The model under review builds one solid part; all positions refer to its coordinate system, in mm. Face numbers are marked on the shaded views. Round coordinates to 2 decimals unless told otherwise and drop trailing zeros. Write each loop counter-clockwise with the first axis right and the second up, starting at its lowest first coordinate (ties: lowest second). Pieces come first, ordered by that corner, then holes.
Item 1: Draft analysis for pull direction Z (two halves, no side actions). For the marked faces 1 and 2, state which applies: +Z half, -Z half, draft (parallel to the pull), parting line (faces both ways), or undercut.
Item 2: To check wall thickness, follow L1, parallel to X at y = 8.6, z = -4; L2, parallel to Z at x = 1, y = 7.35; L3, parallel to X at y = 4.3, z = 0. State the ranges of each line that lie inside material, in increasing order.
Item 3: Add section A-A (y = 7.15). Give the boundary of the cut face in (x, z), plus the area to 3 significant figures.
Item 4: Clearance check with flat-ended pins moving along their axes: pin 1 Ø2.5 at (x, z) = (-0.5, 1) entering from +Y; pin 2 Ø1 at (x, z) = (2.5, 0.5) entering from -Y; pin 3 Ø5 at (x, z) = (-1.5, 2) entering from +Y; pin 4 Ø2 at (y, z) = (5, 1.5) entering from -X. State where each tip first meets the part, or that it passes through.
```python
from build123d import *

# Parameters (mm, degrees)
EXTRUDE_1_DEPTH          = 0.6
EXTRUDE_1_DEPTH_BACK     = 6
SKETCH_5_R               = 0.31
SKETCH_7_R               = 0.28
CUT_EXTRUDE_2_DEPTH      = 16.448840302
CUT_EXTRUDE_3_DEPTH      = 10
CUT_EXTRUDE_3_DEPTH_BACK = 10


with BuildPart() as part:
    # Sketch 2 → Revolve 1 (revolve)
    with BuildSketch(Plane.XY, mode=Mode.PRIVATE) as revolve_1_sk:
        Polygon((0, 0), (-4.618802154, 8), (0, 8), align=None)
    revolve(revolve_1_sk.sketch.rotate(Axis((0, -55.266670228, 0), (0, 1, 0)), 90), axis=Axis((0, -55.266670228, 0), (0, 1, 0)))

    # Sketch 5 → Extrude 1 (add, two sides: drawn at the far end of the back side and taken through both)
    with BuildSketch(Plane(origin=(0, 0, 0), x_dir=(1, 0, 0), z_dir=(0, 1, 0)).offset(-EXTRUDE_1_DEPTH_BACK)):
        with Locations(Location((0, 0, 0), (0, 0, 270))):
            Circle(SKETCH_5_R)
    extrude(amount=EXTRUDE_1_DEPTH + EXTRUDE_1_DEPTH_BACK)

    # Sketch 7 → Cut-Extrude 2 (cut, through all)
    with BuildSketch(Plane.XZ.offset(6)):
        with Locations(Location((0, 0, 0), (0, 0, 270))):
            Circle(SKETCH_7_R)
    extrude(amount=-CUT_EXTRUDE_2_DEPTH, mode=Mode.SUBTRACT)

    # Sketch 4 → Cut-Revolve 2 (revolve, cut)
    with BuildSketch(Plane.XY):
        Polygon((0, 8), (-4.041451884, 8), (0, 1), align=None)
    revolve(axis=Axis((0, 7.19521629, 0), (0, 1, 0)), mode=Mode.SUBTRACT)

    # Sketch 10 → Revolve 3 (revolve)
    with BuildSketch(Plane.XY, mode=Mode.PRIVATE) as revolve_3_sk:
        with BuildLine():
            Line((-4.041451884, 9), (-4.618802154, 9))
            ThreePointArc((-4.618802154, 9), (-5.118802154, 8.5), (-4.618802154, 8))
            Line((-4.618802154, 8), (-4.041451884, 8))
            Line((-4.041451884, 8), (-4.041451884, 9))
        make_face()
    revolve(revolve_3_sk.sketch.rotate(Axis((0, 0, 0), (0, 1, 0)), 270), axis=Axis((0, 0, 0), (0, 1, 0)))

    # Sketch 11 → Cut-Revolve 3 (revolve, cut)
    with BuildSketch(Plane.XY):
        Polygon((-4.041451884, 8), (-4.932498772, 9.543338481), (-1.781160805, 9.543338481), (-1.781160805, 8), align=None)
    revolve(axis=Axis((0, 0, 0), (0, 1, 0)), mode=Mode.SUBTRACT)

    # Sketch 14 → Revolve 4 (revolve)
    with BuildSketch(Plane.XY, mode=Mode.PRIVATE) as revolve_4_sk:
        Polygon((0.325, 3.401430976), (0.325, 3.751430976), (2.165889684, 3.751430976), (1.963817089, 3.401430976), align=None)
    revolve(revolve_4_sk.sketch.rotate(Axis((0, 0, 0), (0, 1, 0)), 270), axis=Axis((0, 0, 0), (0, 1, 0)))

    # Sketch 16 → Cut-Extrude 3 (cut, two sides: drawn at the far end of the back side and taken through both)
    with BuildSketch(Plane.XY.offset(-CUT_EXTRUDE_3_DEPTH_BACK)):
        Polygon((1.38646682, 3.401430976), (4.735566884, 3.401430976), (4.735566884, -6.564906042), (-5.830144142, -6.564906042), (-5.830144142, 3.401430976), align=None)
    extrude(amount=CUT_EXTRUDE_3_DEPTH + CUT_EXTRUDE_3_DEPTH_BACK, mode=Mode.SUBTRACT)

    # Sketch 21 → Revolve 5 (revolve)
    with BuildSketch(Plane.XY, mode=Mode.PRIVATE) as revolve_5_sk:
        Polygon((1.588539414, 3.751430976), (1.588539414, 5.341161575), (1.588539414, 5.501161575), (1.333683802, 5.501161575), (2.805566179, 5.859383166), (2.698088002, 5.673225503), align=None)
    revolve(revolve_5_sk.sketch.rotate(Axis((0, 0.062644637, 0), (0, 1, 0)), 90), axis=Axis((0, 0.062644637, 0), (0, 1, 0)))


solid = part.part
```
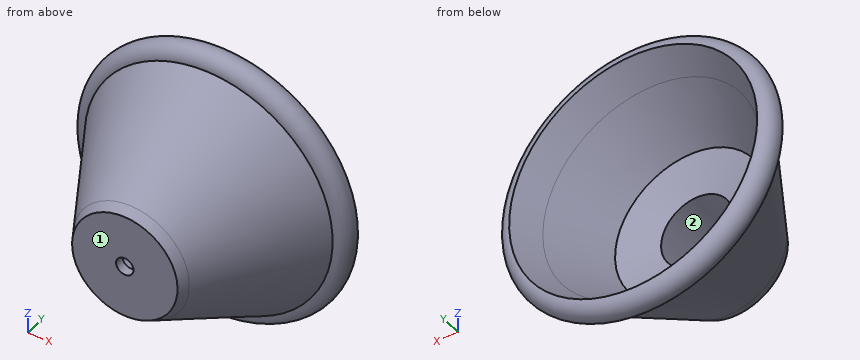
Numbers:
1. face 1: draft
1. face 2: undercut
2. L1: x = -3.18 to -1.8, 1.8 to 3.18
2. L2: z = -4.12 to -3.53, 3.53 to 4.12
2. L3: x = -2.48 to -1.59, 1.59 to 2.48
3. outline: circle Ø8.26 at (0, 0); hole circle Ø7.1 at (0, 0)
3. area: 13.9 mm2
4. pin 1: stops at y = 5.75
4. pin 2: stops at y = 3.55
4. pin 3: stops at y = 9
4. pin 4: stops at x = -3.24
